Read the model definition and answer for the solid it produces. Units are mm, in the model's axes. Give positions to 0.01 mm unless a question says otherwise; leave off trailing zeros. Order: outer loops, then holes, each group sorted by start corner. A loop starts at its lowest first (then second) coordinate and runs counter-clockwise, first axis right, second up. Notation, with made-up numbers: (74.25, 79.25) - (121.25, 79.25) arc R24 cw to (121.25, 112.25) - close; hole circle Ø11 at (45.25, 12). An arc over 180 degrees is marked (long way). Write each question's results on one line, items separated by ' | '. Start each with the question number.
Q1. Find section C-C on x = 0.6. Give the vertices of the cut face in (y, z), and give its area (3 significant figures).
Q2. Flat-ended cylindrical pins translate along their axes: P1, Ø2.5, axis at x = 1, y = 222.5, coming from the -Z side; P2, Ø1.5, axis at x = 0.5, y = 55.5, coming from the +Z side; P3, Ø2.5, axis at x = 1, y = -125.5, coming from the +Z side (3 decimals). Find the tip coordinate at first contact, or state that the pin passes through.
Q3. Find section D-D on y = 127. Give the vertices of the cut face in (x, z), and give its area (3 significant figures).
Q4. Find the intervals of material crossed by line 1 along Z through (x, y) = (-1.2, 203); line 2 along Y through (x, z) = (-0.25, 42); line 3 along Z through (x, y) = (1.7, 20), in increasing order. Write a range as from..to.
Q5. Find section A-A on y = -89. Give the vertices of the cut face in (x, z).
Q6. Find section B-B on z = 50. Give the vertices of the cut face in (x, y), and give its area (3 significant figures).
from build123d import *

# Parameters (mm, degrees)
F1_DEPTH = 2.5
F2_R     = 10
F3_R     = 10


with BuildPart() as f1:
    # F0 (on Right) → F1 (new body, symmetric)
    with BuildSketch(Plane.YZ):
        Polygon((-300, 10), (-300, 0), (-300, -10), (-150, -47.5), (0, -32.5), (300, -32.5), (300, 27.5), (265, 97.5), (175, 97.5), (150, 27.5), (0, 27.5), (-130, 94.5), (-150, 94.5), (-170, 94.5), align=None)
        Polygon((-220, -2.5), (-220, 0), (-220, 2.5), (-100, 2.5), (-80, 2.5), (-80, -2.5), align=None, mode=Mode.SUBTRACT)
        Polygon((270, 2.5), (270, 0), (270, -2.5), (175, -2.5), (175, 2.5), align=None, mode=Mode.SUBTRACT)
        Polygon((-80, 2.5), (-100, 2.5), (-80, -2.5), align=None)
    extrude(amount=F1_DEPTH, both=True)

    # F2
    f2_edges = [f1.edges().sort_by_distance(p)[0] for p in [
        (0, -300, 10),
    ]]
    fillet(f2_edges, radius=F2_R)

    # F3
    f3_edges = [f1.edges().sort_by_distance(p)[0] for p in [
        (0, -300, -10),
    ]]
    fillet(f3_edges, radius=F3_R)


solid = f1.part
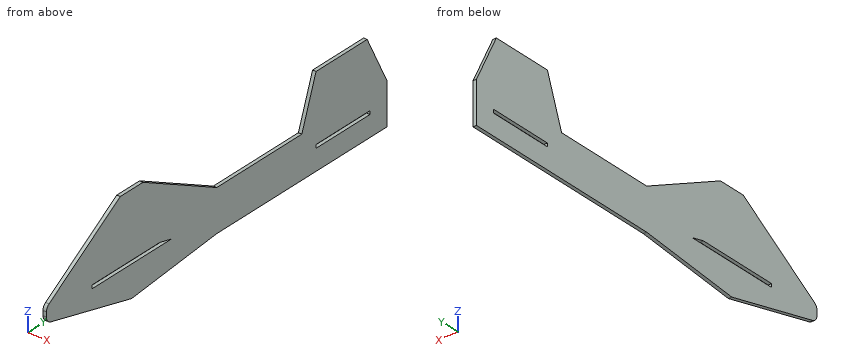
Working result:
1) outline: (-300, -2.19) arc R10 ccw to (-292.43, -11.89) - (-150, -47.5) - (0, -32.5) - (300, -32.5) - (300, 27.5) - (265, 97.5) - (175, 97.5) - (150, 27.5) - (0, 27.5) - (-130, 94.5) - (-170, 94.5) - (-295.45, 12.96) arc R10 ccw to (-300, 4.57) - close; hole (-220, -2.5) - (-80, -2.5) - (-100, 2.5) - (-220, 2.5) - close; hole (175, -2.5) - (270, -2.5) - (270, 2.5) - (175, 2.5) - close | area: 54,100 mm²
2) P1: z = -32.5 | P2: z = 27.5 | P3: z = 92.825
3) outline: (-2.5, -32.5) - (2.5, -32.5) - (2.5, 27.5) - (-2.5, 27.5) - close | area: 300 mm²
4) line 1: -32.5..-2.5, 2.5..97.5 | line 2: -250.77..-28.13, 155.18..292.75 | line 3: -32.5..27.5
5) outline: (-2.5, -41.4) - (2.5, -41.4) - (2.5, -2.5) - (-2.5, -2.5) - close; (-2.5, -0.25) - (2.5, -0.25) - (2.5, 73.37) - (-2.5, 73.37) - close
6) outline: (-2.5, -238.46) - (2.5, -238.46) - (2.5, -43.66) - (-2.5, -43.66) - close; (-2.5, 158.04) - (2.5, 158.04) - (2.5, 288.75) - (-2.5, 288.75) - close | area: 1,630 mm²
